from build123d import *

# Parameters (mm, degrees)
ESQUISSE1_R        = 7.5
ESQUISSE1_R_2      = 2.75
BOSS_EXTRU_1_DEPTH = 15
ESQUISSE2_R        = 7.5
BOSS_EXTRU_2_DEPTH = 2
CONG_1_R           = 1
ESQUISSE3_W        = 1
ESQUISSE3_H        = 1.40589343
BOSS_EXTRU_3_DEPTH = 1
CONG_2_R           = 0.25
CONG_3_R           = 0.25


with BuildPart() as part:
    # Esquisse1 → Boss.-Extru.1 (new body)
    with BuildSketch(Plane.XY):
        Circle(ESQUISSE1_R)
        Circle(ESQUISSE1_R_2, mode=Mode.SUBTRACT)
    extrude(amount=BOSS_EXTRU_1_DEPTH)

    # Esquisse2 → Boss.-Extru.2 (add)
    with BuildSketch(Plane.XY.offset(15)):
        Circle(ESQUISSE2_R)
    extrude(amount=BOSS_EXTRU_2_DEPTH)

    # Congé1
    cong_1_edges = [part.edges().sort_by_distance(p)[0] for p in [
        (-7.5, 0, 17),
    ]]
    fillet(cong_1_edges, radius=CONG_1_R)

    # Esquisse3 → Boss.-Extru.3 (add)
    with BuildSketch(Plane.XY.offset(17)):
        with Locations((0, 5.777793983)):
            Rectangle(ESQUISSE3_W, ESQUISSE3_H)
    extrude(amount=BOSS_EXTRU_3_DEPTH)

    # Congé2
    cong_2_edges = [part.edges().sort_by_distance(p)[0] for p in [
        (-0.5, 6.480740698, 17.5),
        (-0.5, 5.074847268, 17.5),
        (0.5, 5.074847268, 17.5),
        (0.5, 6.480740698, 17.5),
        (-0.5, 5.777793983, 18),
        (0, 5.074847268, 18),
        (0.5, 5.777793983, 18),
        (0, 6.480740698, 18),
    ]]
    fillet(cong_2_edges, radius=CONG_2_R)

    # Congé3
    cong_3_edges = [part.edges().sort_by_distance(p)[0] for p in [
        (0, 6.480740698, 17),
        (-0.5, 5.777793983, 17),
        (0.5, 5.777793983, 17),
        (0, 5.074847268, 17),
        (-0.426776695, 6.407517394, 17),
        (0.426776695, 6.407517394, 17),
        (-0.426776695, 5.148070573, 17),
        (0.426776695, 5.148070573, 17),
    ]]
    fillet(cong_3_edges, radius=CONG_3_R)


solid = part.part
Source: CAD feature listing. Evaluate the final solid. Frame: model axes, mm. Coordinates: 2 decimals unless noted, no trailing zeros. Order: outer loops, then holes, each group sorted by start corner. A loop starts at its lowest first (then second) coordinate and runs counter-clockwise, first axis right, second up. Notation, with made-up numbers: M 27.5,1.25 L 35.5,1.25 A6 ccw 35.5,7.25 Z; hole C -18,-7 d8. An arc over 180 degrees is marked long. Write each question's results on one line, items separated by ' | '. Start each with the question number.
Item 1: First-contact query: pin 1 Ø1.6 at (x, y) = (1, 1) entering from -Z; pin 2 Ø1.5 at (x, z) = (-4.5, 7.5) entering from +Y; pin 3 Ø5 at (x, z) = (6, 9.5) entering from -Y. Flat tips, straight axial feed; report the tip coordinate or a pass-through.
Item 2: Cut plane B-B (z = 6.5). Return loops of the section in (x, y), and give its area (3 significant figures).
Item 3: Draft query along Y for faces 1 (the face through (3, 0, 0)), 2 (the face through (-0.596, -2.685, 7.395)), 3 (the face through (-7.493, 0.33, 7.888)). Return one class per face: pulls with the +Y half, pulls with the -Y half, needs draft (parallel to the pull), parting line crosses it, or undercut.
Item 4: Line query: probe 1 along Y at (x, z) = (0, 8.5); probe 2 along Z at (x, y) = (-1, 2.75); probe 3 along Z at (x, y) = (0.5, 0). Output: solid intervals per line, ascending.
Item 5: Cut plane A-A (y = 0). Return loops of the section in (x, z), and give its area (3 significant figures).
Checked values:
1) pin 1: stops at z = 15 | pin 2: stops at y = 6.5 | pin 3: stops at y = -6.63
2) outline: C 0,0 d15; hole C 0,0 d5.5 | area: 153 mm2
3) face 1: needs draft | face 2: undercut | face 3: parting line crosses it
4) probe 1: y = -7.5 to -2.75, 2.75 to 7.5 | probe 2: z = 0 to 17 | probe 3: z = 15 to 17
5) outline: M -7.5,0 L -2.75,0 L -2.75,15 L 2.75,15 L 2.75,0 L 7.5,0 L 7.5,16 A1 ccw 6.5,17 L -6.5,17 A1 ccw -7.5,16 Z | area: 172 mm2
